```python
from build123d import *

# Parameters (mm, degrees)
SKETCH_1_W        = 1000
SKETCH_1_H        = 80
EXTRUDE_1_DEPTH   = 20
SKETCH_2_W        = 20
SKETCH_2_H        = 80
EXTRUDE_1_2_DEPTH = 80
SKETCH_3_R        = 35
EXTRUDE_2_DEPTH   = 980


with BuildPart() as part:
    # 草图1 → Extrude 1 (new body)
    with BuildSketch(Plane(origin=(0, 0, 0), x_dir=(0, 0, -1), z_dir=(1, 0, 0))):
        Rectangle(SKETCH_1_W, SKETCH_1_H)
    extrude(amount=EXTRUDE_1_DEPTH)

    # 草图2 → Extrude 1 2 (add)
    with BuildSketch(Plane(origin=(20, 0, 0), x_dir=(0, 0, -1), z_dir=(1, 0, 0))):
        with Locations((-490, 0)):
            Rectangle(SKETCH_2_W, SKETCH_2_H)
    extrude_1_2 = extrude(amount=EXTRUDE_1_2_DEPTH)

    # 镜向1: Extrude 1 2 across plane
    add(extrude_1_2.mirror(Plane.XY))

    # 草图3 → 凸台-拉伸2 (add)
    with BuildSketch(Plane.XY.offset(500)):
        with Locations((60, 0)):
            Circle(SKETCH_3_R)
    extrude(amount=-EXTRUDE_2_DEPTH)


solid = part.part
```
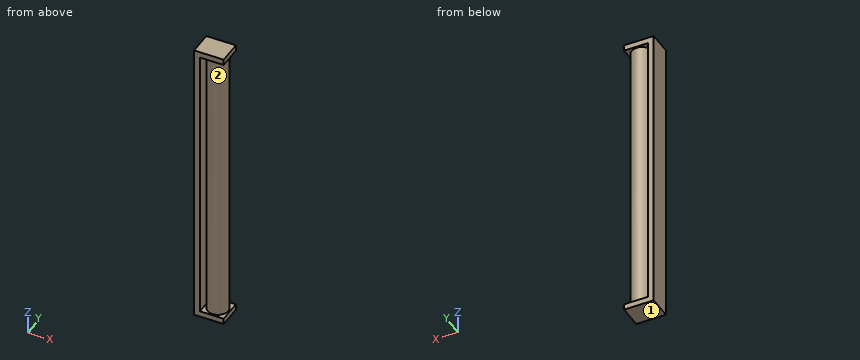
Here's how the part is built. I have some questions about the finished solid (model axes, mm). Face numbers are marked on the shaded views. Give positions to 0.01 mm unless a question says otherwise; leave off trailing zeros. Order: outer loops, then holes, each group sorted by start corner. A loop starts at its lowest first (then second) coordinate and runs counter-clockwise, first axis right, second up. Notation, with made-up numbers: (-6.5, 72) - (15.5, 72) arc R23 ccw to (15.5, 100) - close; hole circle Ø1 at (-39, -15.5). An arc over 180 degrees is marked (long way). Answer as a JSON object with one key per item and string values. Group by question number.
Item 1: If we mould it in two halves opening along X, with no side actions, what happens to the marked faces 1 and 2? For each: pulls with the +X half, pulls with the -X half, needs draft (parallel to the pull), parting line crosses it, or undercut.
Item 2: If we section it at B-B on z = -29.5: Please give me the cut outline in (x, y).
Item 3: If we section it at A-A on y = 0: Please give me the cut outline in (x, z).
Item 4: Please list where these lines run through material, in increasing order: probe 1 along Z at (x, y) = (33.5, 35); probe 2 along Y at (x, z) = (61.5, -195); probe 3 along X at (y, z) = (-11, 247).
Item 5: If we section it at C-C on x = 60: Please give me the cut outline in (y, z).
Item 6: For P1, Ø8, axis at y = -15, z = 358, coming from the +X side; P2, Ø2, axis at x = 45, z = -213.5, coming from the -Y side; P3, Ø12, axis at x = 29.5, z = 158.5, coming from the -Y side (3 decimals), each with a flat end and sliding along its axis, tell me the tip position at first contact or that it passes through.
Result set:
{
 "1": {"face 1": "needs draft", "face 2": "undercut"},
 "2": {"outline": "(0, -40) - (20, -40) - (20, 40) - (0, 40) - close; circle Ø70 at (60, 0)"},
 "3": {"outline": "(0, -500) - (100, -500) - (100, -480) - (95, -480) - (95, 480) - (100, 480) - (100, 500) - (0, 500) - close; hole (20, -480) - (25, -480) - (25, 480) - (20, 480) - close"},
 "4": {"probe 1": "-500 to -480, 480 to 500", "probe 2": "-34.97 to 34.97", "probe 3": "0 to 20, 26.77 to 93.23"},
 "5": {"outline": "(-40, -500) - (40, -500) - (40, -480) - (35, -480) - (35, 480) - (40, 480) - (40, 500) - (-40, 500) - (-40, 480) - (-35, 480) - (-35, -480) - (-40, -480) - close"},
 "6": {"P1": "x = 93.23", "P2": "y = -32.08", "P3": "y = -24.995"}
}
